```python
from build123d import *

# Parameters (mm, degrees)
SKETCH1_R           = 45
BOSS_EXTRUDE1_DEPTH = 4
SKETCH2_R           = 42.5
BOSS_EXTRUDE2_DEPTH = 4.2
SKETCH4_R           = 13
CUT_EXTRUDE1_DEPTH  = 65.165722937
SKETCH5_W           = 46
SKETCH5_H           = 61
CUT_EXTRUDE2_DEPTH  = 4


with BuildPart() as part:
    # Sketch1 → Boss-Extrude1 (new body)
    with BuildSketch(Plane.XY):
        Circle(SKETCH1_R)
    extrude(amount=BOSS_EXTRUDE1_DEPTH)

    # Sketch2 → Boss-Extrude2 (add)
    with BuildSketch(Plane.XY.offset(4)):
        Circle(SKETCH2_R)
    extrude(amount=BOSS_EXTRUDE2_DEPTH)

    # Sketch4 → Cut-Extrude1 (cut, through all)
    with BuildSketch(Plane.XY.offset(8.2)):
        Circle(SKETCH4_R)
    extrude(amount=-CUT_EXTRUDE1_DEPTH, mode=Mode.SUBTRACT)

    # Sketch5 → Cut-Extrude2 (cut)
    with BuildSketch(Plane(origin=(0, 0, 0), x_dir=(-1, 0, 0), z_dir=(0, 0, -1))):
        Rectangle(SKETCH5_W, SKETCH5_H)
    extrude(amount=-CUT_EXTRUDE2_DEPTH, mode=Mode.SUBTRACT)


solid = part.part
```
Build history of the part. All positions in model axes, mm. A direction names the side the tool comes from. Round coordinates to 2 decimals unless told otherwise and drop trailing zeros. Order: outer loops, then holes, each group sorted by start corner. A loop starts at its lowest first (then second) coordinate and runs counter-clockwise, first axis right, second up. Notation, with made-up numbers: (41, -23) - (69, -23) arc R20 ccw to (69, 3) - close; hole circle Ø3 at (23, 5.5). An arc over 180 degrees is marked (long way). Use a Markdown table: item, result.
1) Saw through at C-C on z = 2. Write the cut outline in (x, y).
Recorded:
| item | result |
|---|---|
| outline | circle Ø90 at (0, 0); hole (-23, -30.5) - (23, -30.5) - (23, 30.5) - (-23, 30.5) - close |
2) Saw through at D-D on x = -16.5. Write the cut outline in (y, z).
Recorded:
| item | result |
|---|---|
| outline | (-41.87, 0) - (-30.5, 0) - (-30.5, 4) - (30.5, 4) - (30.5, 0) - (41.87, 0) - (41.87, 4) - (39.17, 4) - (39.17, 8.2) - (-39.17, 8.2) - (-39.17, 4) - (-41.87, 4) - close |
3) Saw through at B-B on x = 0. Write the cut outline in (y, z).
Recorded:
| item | result |
|---|---|
| outline | (-45, 0) - (-30.5, 0) - (-30.5, 4) - (-13, 4) - (-13, 8.2) - (-42.5, 8.2) - (-42.5, 4) - (-45, 4) - close; (13, 4) - (30.5, 4) - (30.5, 0) - (45, 0) - (45, 4) - (42.5, 4) - (42.5, 8.2) - (13, 8.2) - close |
4) Saw through at A-A on y = 0. Write the cut outline in (x, z).
Recorded:
| item | result |
|---|---|
| outline | (-45, 0) - (-23, 0) - (-23, 4) - (-13, 4) - (-13, 8.2) - (-42.5, 8.2) - (-42.5, 4) - (-45, 4) - close; (13, 4) - (23, 4) - (23, 0) - (45, 0) - (45, 4) - (42.5, 4) - (42.5, 8.2) - (13, 8.2) - close |
5) Wall check: L1, parallel to Y at x = 0, z = 7.15; L2, parallel to Z at x = -12.5, y = 28.5; L3, parallel to Y at x = 4.5, z = 3.5. Give the ranges that are in metal, low to high.
Recorded:
| item | result |
|---|---|
| L1 | y = -42.5 to -13, 13 to 42.5 |
| L2 | z = 4 to 8.2 |
| L3 | y = -44.77 to -30.5, 30.5 to 44.77 |
6) Flat gauge pins, fed straight in: pin 1 Ø3 at (x, z) = (8.5, 3.5) entering from +Y; pin 2 Ø3 at (y, z) = (-2.5, 3) entering from -X; pin 3 Ø12 at (x, y) = (15, -14) entering from -Z; pin 4 Ø12 at (x, y) = (-28, -33) entering from +Z. Where does each tip first touch, or does it go through?
Recorded:
| item | result |
|---|---|
| pin 1 | stops at y = 44.45 |
| pin 2 | stops at x = -44.99 |
| pin 3 | stops at z = 4 |
| pin 4 | stops at z = 8.2 |
7) Pull direction Y, two halves, no side cores. Call faces 1 (the face through (0, -30.5, 2)), 2 (the face through (-33.727, -25.861, 6.071)), 3 (the face through (-10, -9, 8.2)): pulls with the +Y half, pulls with the -Y half, needs draft (parallel to the pull), parting line crosses it, or undercut.
Recorded:
| item | result |
|---|---|
| face 1 | undercut |
| face 2 | parting line crosses it |
| face 3 | needs draft |
8) Tool access for faces 4 (the face through (-10.316, -7.91, 6.129)), 5 (the face through (-23, 0, 2)), 6 (the face through (-26.9, -33.1, 4)): list every direction of +Z, -Z, +X, -X, +Y, -Y with a clear straight run to the whole face (end or side of a thin tool).
Recorded:
| item | result |
|---|---|
| face 4 | +Z, -Z |
| face 5 | -Z |
| face 6 | +Z |
